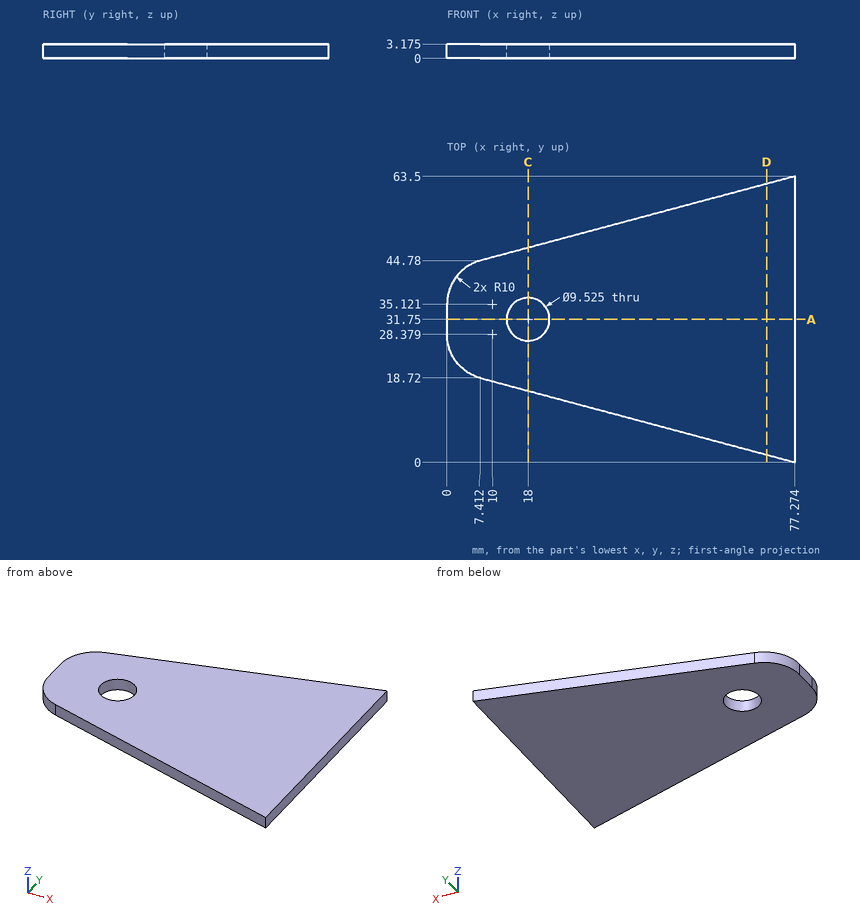
Print and shaded views of the part. All mm, measured from the part's lowest x, y and z. Give positions to 0.01 mm unless a question says otherwise; leave off trailing zeros. Loops run counter-clockwise (first coordinate to the right, second up) from the corner with the lowest first, then second, coordinate; pieces in that order, holes last. Notation, with made-up numbers: M 69,16 L 109,16 A20 ccw 109,34 Z; hole C -1.5,89.5 d3. An arc over 180 degrees is marked long. Write each question's results on one line, items separated by ' | '.
Q1. Band-saw the part on C-C on x = 18. Write the cut outline in (y, z) (1 decimal).
Geometry check:
outline: M 15.9,0 L 27,0 L 27,3.2 L 15.9,3.2 Z; M 36.5,0 L 47.6,0 L 47.6,3.2 L 36.5,3.2 Z
Q2. Probe probe 1 along Y at (x, z) = (18, 1.25); probe 2 along X at (y, z) = (35.5, 1.25) (1 decimal); probe 3 along Y at (x, z) = (34.5, 0.25). List the from-to ranges inside material, lowest first.
Geometry check:
probe 1: y = 15.88 to 26.99, 36.51 to 47.62 | probe 2: x = 0 to 15.1, 20.9 to 77.3 | probe 3: y = 11.46 to 52.04
Q3. Band-saw the part on A-A on y = 31.75. Write the cut outline in (x, z) (1 decimal).
Geometry check:
outline: M 0,0 L 13.2,0 L 13.2,3.2 L 0,3.2 Z; M 22.8,0 L 77.3,0 L 77.3,3.2 L 22.8,3.2 Z
Q4. Band-saw the part on D-D on x = 71. Write the cut outline in (y, z) (1 decimal), and give its area (3 significant figures).
Geometry check:
outline: M 1.7,0 L 61.8,0 L 61.8,3.2 L 1.7,3.2 Z | area: 191 mm²
Q5. Flat gauge pin, fed straight in: P1, Ø1, axis at x = 22, z = 1.5, coming from the -Y side. Where does the tip first touch, or does it go through?
Geometry check:
P1: stops at y = 14.68
